```python
from build123d import *

# Parameters (mm, degrees)
F0_R     = 21.336
F0_R_2   = 19.685
F1_DEPTH = 1.27
F2_DEPTH = 6.35
F3_R     = 6.35


with BuildPart() as f1:
    # F0 (on Top) → F1 (new body)
    with BuildSketch(Plane.XY):
        Circle(F0_R)
        Circle(F0_R_2, mode=Mode.SUBTRACT)
    extrude(amount=F1_DEPTH)

    # F0 (on Top) → F2 (join)
    with BuildSketch(Plane.XY):
        with BuildLine():
            ThreePointArc((23.9050999455, -6.4692674698), (24.5490837421, -3.2630832697), (24.765, 0))
            ThreePointArc((24.765, 0), (19.6285885254, 15.1004548773), (6.35, 23.9370575677))
            ThreePointArc((6.35, 23.9370575677), (4.0651088886, 24.4290833787), (1.7440091422, 24.703515076))
            ThreePointArc((1.7440091422, 24.703515076), (1.8643178935, 24.3286489263), (1.905, 23.9370575677))
            ThreePointArc((1.905, 23.9370575677), (-0.3915913586, 22.0727396742), (-1.7440091422, 24.703515076))
            ThreePointArc((-1.7440091422, 24.703515076), (-4.0651088886, 24.4290833787), (-6.35, 23.9370575677))
            ThreePointArc((-6.35, 23.9370575677), (-21.4471191247, 12.3825), (-23.9050999455, -6.4692674698))
            ThreePointArc((-23.9050999455, -6.4692674698), (-23.1887612414, -8.6940541227), (-22.2658761897, -10.8414013165))
            ThreePointArc((-22.2658761897, -10.8414013165), (-20.1370690632, -10.1581864481), (-18.8250999455, -11.9685287839))
            ThreePointArc((-18.8250999455, -11.9685287839), (-19.3113489683, -13.239815795), (-20.5218670475, -13.8621137596))
            ThreePointArc((-20.5218670475, -13.8621137596), (-19.1236523528, -15.735029256), (-17.5550999455, -17.4677900979))
            ThreePointArc((-17.5550999455, -17.4677900979), (0, -24.765), (17.5550999455, -17.4677900979))
            ThreePointArc((17.5550999455, -17.4677900979), (19.1236523528, -15.735029256), (20.5218670475, -13.8621137596))
            ThreePointArc((20.5218670475, -13.8621137596), (19.0803215513, -11.0160287839), (22.2658761897, -10.8414013165))
            ThreePointArc((22.2658761897, -10.8414013165), (23.1887612414, -8.6940541227), (23.9050999455, -6.4692674698))
        make_face()
        Circle(F0_R, mode=Mode.SUBTRACT)
        with BuildLine():
            ThreePointArc((1.7440091422, 24.703515076), (4.0651088886, 24.4290833787), (6.35, 23.9370575677))
            ThreePointArc((6.35, 23.9370575677), (0, 30.2870575677), (-6.35, 23.9370575677))
            ThreePointArc((-6.35, 23.9370575677), (-4.0651088886, 24.4290833787), (-1.7440091422, 24.703515076))
            ThreePointArc((-1.7440091422, 24.703515076), (0, 25.8420575677), (1.7440091422, 24.703515076))
        make_face()
        with BuildLine():
            ThreePointArc((17.5550999455, -17.4677900979), (26.2293612595, -15.1435287839), (23.9050999455, -6.4692674698))
            ThreePointArc((23.9050999455, -6.4692674698), (23.1887612414, -8.6940541227), (22.2658761897, -10.8414013165))
            ThreePointArc((22.2658761897, -10.8414013165), (22.5404422812, -11.3754979015), (22.6350999455, -11.9685287839))
            ThreePointArc((22.6350999455, -11.9685287839), (22.0013869566, -13.3872797611), (20.5218670475, -13.8621137596))
            ThreePointArc((20.5218670475, -13.8621137596), (19.1236523528, -15.735029256), (17.5550999455, -17.4677900979))
        make_face()
        with BuildLine():
            ThreePointArc((-22.2658761897, -10.8414013165), (-23.1887612414, -8.6940541227), (-23.9050999455, -6.4692674698))
            ThreePointArc((-23.9050999455, -6.4692674698), (-26.2293612595, -15.1435287839), (-17.5550999455, -17.4677900979))
            ThreePointArc((-17.5550999455, -17.4677900979), (-19.1236523528, -15.735029256), (-20.5218670475, -13.8621137596))
            ThreePointArc((-20.5218670475, -13.8621137596), (-22.3798783397, -12.9210287839), (-22.2658761897, -10.8414013165))
        make_face()
    extrude(amount=F2_DEPTH)

    # F3
    f3_edges = [f1.edges().sort_by_distance(p)[0] for p in [
        (6.35, 23.937058, 3.175),
        (-23.9051, -6.469267, 3.175),
        (17.5551, -17.46779, 3.175),
        (23.9051, -6.469267, 3.175),
        (-6.35, 23.937058, 3.175),
        (-17.5551, -17.46779, 3.175),
    ]]
    fillet(f3_edges, radius=F3_R)


solid = f1.part
```
Verification items for the finished model (mm, model axes). A direction names the side the tool comes from. Give positions to 0.01 mm unless a question says otherwise; leave off trailing zeros. Loops run counter-clockwise (first coordinate to the right, second up) from the corner with the lowest first, then second, coordinate; pieces in that order, holes last. Notation, with made-up numbers: M -21.5,28.5 L 2.5,28.5 A16 cw 2.5,52.5 Z; hole C 18,-36 d8. An arc over 180 degrees is marked long. One line per question, with ' | ' between items.
Item 1: Section check D-D, the plane y = 20.5. Record the cut outline in (x, z), plus the area to 3 significant figures.
Completed:
outline: M -13.89,0 L 13.89,0 L 13.89,6.35 L 5.91,6.35 L 5.91,1.27 L -5.91,1.27 L -5.91,6.35 L -13.89,6.35 Z | area: 116 mm^2
Item 2: Thickness scan on line 1 (Y direction, x = 19.5, z = 3.5); line 2 (Z direction, x = -12, y = 17.5); line 3 (X direction, y = 15.5, z = 0.5). Record the ranges inside material, lowest first. Write a range as [from, to].
Completed:
line 1: y = [-18.23, -13.42], [-10.51, -8.66], [8.66, 15.27] | line 2: z = [0, 1.27] | line 3: x = [-19.31, -12.13], [12.13, 19.31]
Item 3: Section check A-A, the plane x = 0. Record the cut outline in (y, z) (3 decimals).
Completed:
outline: M -24.765,0 L -19.685,0 L -19.685,1.27 L -21.336,1.27 L -21.336,6.35 L -24.765,6.35 Z; M 19.685,0 L 22.032,0 L 22.032,6.35 L 21.336,6.35 L 21.336,1.27 L 19.685,1.27 Z; M 25.842,0 L 30.287,0 L 30.287,6.35 L 25.842,6.35 Z
Item 4: Section check C-C, the plane x = 12. Record the cut outline in (y, z).
Completed:
outline: M -21.66,0 L -15.6,0 L -15.6,1.27 L -17.64,1.27 L -17.64,6.35 L -21.66,6.35 Z; M 15.6,0 L 21.66,0 L 21.66,6.35 L 17.64,6.35 L 17.64,1.27 L 15.6,1.27 Z
Item 5: Tool access check on faces 1 (the face through (9.845, -18.929, 3.774)), 2 (the face through (0.105, 30.286, 3.131)). Record the directions out of +Z, -Z, +X, -X, +Y, -Y that give a thin tool (end or side, any length) a straight path to the whole face; none if there is none.
Completed:
face 1: +Z | face 2: +Z, -Z, +Y
Item 6: Draft check along Y on faces 3 (the face through (-15.62, -11.98, 0.63)), 4 (the face through (-0.229, -24.764, 3.131)), 5 (the face through (6, -19, 1.27)), 6 (the face through (-4.1, 21.2, 6.35)). Enter one of: +Y half, -Y half, draft (parallel to the pull), parting line (faces both ways), or undercut.
Completed:
face 3: undercut | face 4: -Y half | face 5: undercut | face 6: draft
Item 7: Section check B-B, the plane y = -16.5. Record the cut outline in (x, z).
Completed:
outline: M -25.18,0 L -10.74,0 L -10.74,1.27 L -13.53,1.27 L -13.53,6.35 L -25.18,6.35 Z; M 10.74,0 L 25.18,0 L 25.18,6.35 L 13.53,6.35 L 13.53,1.27 L 10.74,1.27 Z
Item 8: Depth check by flat-ended pin: P1, Ø3, axis at x = -18.5, z = 2, coming from the +Y side; P2, Ø2, axis at y = 17, z = 5.5, coming from the -X side. Enter the tip coordinate at first touch or a pass-through.
Completed:
P1: stops at y = 18.01 | P2: stops at x = -18.9
